Autodesk Inventor part; units mm, degrees
sketch "Sketch1" plane through (0, 0, 0) normal (0, 1, 0) x (-1, 0, 0)
  point P0 (0, 0)
sketch "Sketch2" plane through (0, 0, 0) normal (0, 1, 0) x (-1, 0, 0)
  point P0 (0, 0)
sketch "Sketch3" plane through (0, 0, 0) normal (0, 1, 0) x (-1, 0, 0)
  line L0 (93.3518, 235.1866) -> (-3.1482, 235.1866)
  line L1 (-3.1482, 235.1866) -> (-3.1482, -6.0634)
  line L2 (-3.1482, -6.0634) -> (93.3518, -6.0634)
  line L3 (93.3518, -6.0634) -> (93.3518, 235.1866)
  point P0 (0, 0)
  dimension "d0" = 241.25
  dimension "d1" = 96.5
extrude "Extrusion1" add sketch "Sketch3" along normal blind 30
sketch "Sketch4" plane through (0, 0, 0) normal (0, -1, 0) x (1, 0, 0)
  line L0 (-93.3518, -6.0634) -> (-93.3518, 235.1866)
  line L1 (-93.3518, 82.5616) -> (3.1482, 82.5616)
  line L2 (3.1482, 82.5616) -> (3.1482, 146.5616)
  line L3 (3.1482, 146.5616) -> (-93.3518, 146.5616)
  line L4 (-93.3518, 146.5616) -> (-93.3518, 82.5616)
  point P0 (0, 0)
  point P1 (-93.3518, 114.5616)
  point P2 (-93.3518, 114.5616)
  dimension "d4" = 64
  dimension "d5" = 0
  dimension "d6" = 96.5
  dimension "d7" = 0
extrude "Extrusion2" cut sketch "Sketch4" against normal blind 28
sketch "Sketch5" plane through (0, 0, 0) normal (0, -1, 0) x (1, 0, 0)
  line L0 (3.1482, 82.5616) -> (-93.3518, 82.5616)
  line L1 (-93.3518, -6.0634) -> (-93.3518, 82.5616)
  line L2 (3.1482, -6.0634) -> (-93.3518, -6.0634)
  line L3 (3.1482, 82.5616) -> (3.1482, -6.0634)
  line L4 (-93.3518, 146.5616) -> (3.1482, 146.5616)
  line L5 (3.1482, 235.1866) -> (3.1482, 146.5616)
  line L6 (-93.3518, 235.1866) -> (3.1482, 235.1866)
  line L7 (-93.3518, 146.5616) -> (-93.3518, 235.1866)
  line L8 (-91.3518, 80.5616) -> (1.1482, 80.5616)
  line L9 (1.1482, 80.5616) -> (1.1482, -4.0634)
  line L10 (1.1482, -4.0634) -> (-91.3518, -4.0634)
  line L11 (-91.3518, -4.0634) -> (-91.3518, 80.5616)
  line L12 (-91.3518, 233.1866) -> (1.1482, 233.1866)
  line L13 (1.1482, 233.1866) -> (1.1482, 148.5616)
  line L14 (1.1482, 148.5616) -> (-91.3518, 148.5616)
  line L15 (-91.3518, 148.5616) -> (-91.3518, 233.1866)
  point P0 (0, 0)
  dimension "d10" = 2
  dimension "d11" = 2
extrude "Extrusion3" cut sketch "Sketch5" against normal blind 28 contours L8 L9 L10 L11 | L12 L13 L14 L15
sketch "Sketch6" plane through (-93.3518, 0, 235.1866) normal (-1, 0, 0) x (0, 0, 1)
  point P0 (-235.1866, 0)
  point P1 (-196.9375, 14)
sketch "Sketch7" plane through (-91.3518, 0, 148.5616) normal (0, 0, 1) x (1, 0, 0)
  line L0 (92.5, 0) -> (0, 0)
  line L1 (92.5, 0) -> (92.5, 28)
  line L2 (92.5, 28) -> (0, 28)
  line L3 (0, 0) -> (0, 28)
  point P0 (91.3518, 0)
sketch "Sketch9" plane through (3.1482, 0, -6.0634) normal (1, 0, 0) x (0, 0, -1)
  line L0 (-152.625, 28) -> (-152.625, 26)
  line L1 (-152.625, 0) -> (-152.625, 28)
  line L2 (-152.625, 0) -> (-152.625, 4)
  line L3 (-152.625, 4) -> (-155.625, 4)
  line L4 (-155.625, 4) -> (-155.625, 26)
  line L5 (-155.625, 26) -> (-152.625, 26)
  line L6 (-152.625, 26) -> (-152.625, 4)
  line L7 (-88.625, 28) -> (-152.625, 28)
  line L8 (-120.625, 28) -> (-120.625, 0)
  line L9 (-88.625, 0) -> (-88.625, 28)
  line L10 (-88.625, 4) -> (-85.625, 4)
  line L11 (-85.625, 4) -> (-85.625, 26)
  line L12 (-85.625, 26) -> (-88.625, 26)
  line L13 (-88.625, 26) -> (-88.625, 4)
  line L14 (-152.625, 28) -> (-157.625, 28)
  line L15 (-157.625, 28) -> (-157.625, 2)
  line L16 (-157.625, 2) -> (-152.625, 2)
  line L17 (-88.625, 28) -> (-83.625, 28)
  line L18 (-83.625, 28) -> (-83.625, 2)
  line L19 (-83.625, 2) -> (-88.625, 2)
  line L20 (-152.625, 26) -> (-152.625, 28)
  line L21 (-154.625, 0) -> (-154.625, 28)
  line L22 (-152.625, 2) -> (-152.625, 4)
  line L23 (-152.625, 26) -> (-152.625, 4)
  line L24 (-88.625, 2) -> (-88.625, 4)
  line L25 (-88.625, 0) -> (-88.625, 28)
  line L26 (-88.625, 4) -> (-88.625, 26)
  line L27 (-88.625, 28) -> (-88.625, 26)
  point P0 (-6.0634, 0)
  dimension "d28" = 2
  dimension "d29" = 4
  dimension "d30" = 3
  dimension "d31" = 2
  dimension "d36" = 22
  dimension "d37" = 2
  dimension "d38" = 5
extrude "Extrusion5" add sketch "Sketch9" against normal up to surface (96.5 mm away) contours L17 L18 L19 L9 L10 L11 L12 | L0 L5 L21 L14 | L21 L5 L4 L3 L16 L15 L14 | L1 L16 L21 L3
extrude "Extrusion6" cut sketch "Sketch9" against normal blind 94.5 contours L1 L3 L21 L5 | L21 L3 L4 L5 | L12 L11 L10 L9
sketch "Sketch11" plane through (3.1482, 4, 149.5616) normal (0, 0, -1) x (-1, 0, 0)
  point P0 (3.1482, -4)
properties part number "kontroller"
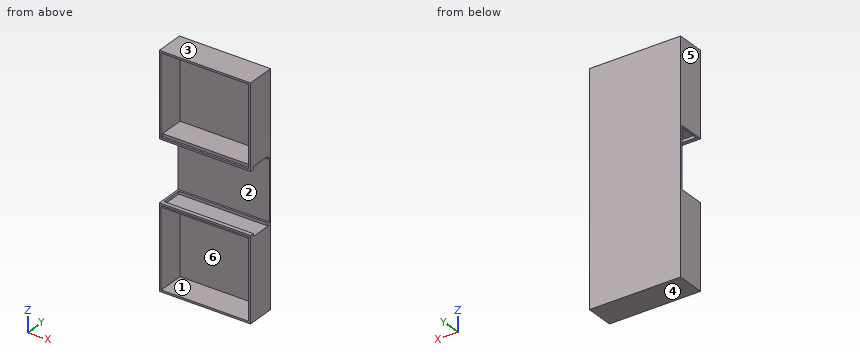
Geometry check sheet. Reference: the model listing, model coordinates, mm. Face numbers are marked on the shaded views. A direction names the side the tool comes from. Round coordinates to 2 decimals unless told otherwise and drop trailing zeros. Write each loop counter-clockwise with the first axis right and the second up, starting at its lowest first coordinate (ties: lowest second). Pieces come first, ordered by that corner, then holes. Notation, with made-up numbers: (74.5, 89) - (101.5, 89) arc R19 ccw to (101.5, 93) - close; hole circle Ø7 at (32, 35.25). An arc over 180 degrees is marked (long way). Write each question's results on one line, items separated by ' | '.
(1) Sectioned sample at B-B, the plane z = 61. Enter the section's corners in (x, y), plus the area to 3 significant figures.
Computed:
outline: (-93.35, 0) - (-91.35, 0) - (-91.35, 28) - (1.15, 28) - (1.15, 0) - (3.15, 0) - (3.15, 30) - (-93.35, 30) - close | area: 305 mm^2
(2) Sectioned sample at C-C, the plane x = -54. Enter the section's corners in (y, z).
Computed:
outline: (0, -6.06) - (30, -6.06) - (30, 235.19) - (0, 235.19) - (0, 233.19) - (28, 233.19) - (28, 151.56) - (2, 151.56) - (2, 148.56) - (0, 148.56) - (0, 146.56) - (4, 146.56) - (4, 149.56) - (26, 149.56) - (26, 146.56) - (28, 146.56) - (28, 82.56) - (26, 82.56) - (26, 79.56) - (4, 79.56) - (4, 82.56) - (0, 82.56) - (0, 80.56) - (2, 80.56) - (2, 77.56) - (28, 77.56) - (28, -4.06) - (0, -4.06) - close
(3) Draft check along X on the marked faces 4, 5 and 6. Enter one of: pulls with the +X half, pulls with the -X half, needs draft (parallel to the pull), parting line crosses it, or undercut.
Computed:
face 4: needs draft | face 5: pulls with the -X half | face 6: undercut
(4) Set-up check for the marked faces 1, 2 and 3: record each of +Z, -Z, +X, -X, +Y, -Y from which the full face is reachable in a straight line by a thin tool's end or side.
Computed:
face 1: -Y | face 2: +X, -X, -Y | face 3: +Z, +X, -X, +Y, -Y
(5) Thickness scan on probe 1 along Z at (x, y) = (-39, 8.75); probe 2 along Z at (x, y) = (-61, 26.5); probe 3 along X at (y, z) = (2, 30). Record the ranges inside material, lowest first. Write a range as from..to.
Computed:
probe 1: z = -6.06..-4.06, 77.56..79.56, 149.56..151.56, 233.19..235.19 | probe 2: z = -6.06..-4.06, 77.56..82.56, 146.56..151.56, 233.19..235.19 | probe 3: x = -93.35..-91.35, 1.15..3.15
(6) Sectioned sample at A-A, the plane y = 23.75. Enter the section's corners in (x, z), plus the area to 3 significant figures.
Computed:
outline: (-93.35, -6.06) - (3.15, -6.06) - (3.15, 79.56) - (-91.35, 79.56) - (-91.35, 82.56) - (-93.35, 82.56) - close; (-93.35, 146.56) - (-91.35, 146.56) - (-91.35, 149.56) - (3.15, 149.56) - (3.15, 235.19) - (-93.35, 235.19) - close; hole (-91.35, -4.06) - (1.15, -4.06) - (1.15, 77.56) - (-91.35, 77.56) - close; hole (-91.35, 151.56) - (1.15, 151.56) - (1.15, 233.19) - (-91.35, 233.19) - close | area: 1,440 mm^2
(7) Depth check by flat-ended pin: pin 1 Ø1.5 at (x, z) = (-35.5, 150.5) entering from -Y; pin 2 Ø0.9 at (y, z) = (12.5, 81) entering from +X; pin 3 Ø19 at (x, z) = (-28, 99) entering from -Y. Enter the tip coordinate at first touch or a pass-through.
Computed:
pin 1: stops at y = 2 | pin 2: stops at x = -91.35 | pin 3: stops at y = 28
